from build123d import *

# Parameters (mm, degrees)
F0_W            = 17.96984524
F0_H            = 38.1
F3_DEPTH        = 25.4
F3_COPIES_COUNT = 10


# Not quite as in the source:
# - a pattern or mirror of a feature is missing from the dataset's text; its kind, count and spacing are read off the source's solid


with BuildPart() as f1:
    # F0 (on Front) → F1 (revolve)
    with BuildSketch(Plane.XZ):
        with Locations((-8.98492262, 22.0940720202)):
            Rectangle(F0_W, F0_H)
    revolve(axis=Axis((-8.98492262, 0, 3.0440720202), (1, 0, 0)))

    # F2 (on face) → F3 (cut)
    with BuildSketch(Plane.YZ):
        with BuildLine():
            Line((-6.214665944, 40.6338036926), (-4.1235210374, 31.6734537482))
            Line((-4.1235210374, 31.6734537482), (0, 31.6734537482))
            Line((0, 31.6734537482), (0, 41.1440720202))
            ThreePointArc((0, 41.1440720202), (-3.117789544, 41.0162906591), (-6.214665944, 40.6338036926))
        make_face()
        with BuildLine():
            Line((0, 41.1440720202), (0, 31.6734537482))
            Line((0, 31.6734537482), (4.2036371306, 31.6734537482))
            Line((4.2036371306, 31.6734537482), (6.1898369976, 40.6379002098))
            ThreePointArc((6.1898369976, 40.6379002098), (3.1052492637, 41.0173182208), (0, 41.1440720202))
        make_face()
    f3 = extrude(amount=-F3_DEPTH, mode=Mode.SUBTRACT)

    # F3_copies: F3 ×10 about axis
    f3_copies_axis = Axis((0, 0, 3.044072), (1, 0, 0))
    for i in range(1, F3_COPIES_COUNT):
        add(f3.rotate(f3_copies_axis, i * 360 / F3_COPIES_COUNT), mode=Mode.SUBTRACT)


solid = f1.part
Input: part model. Units: mm. Frame: model coordinates. A direction names the side the tool comes from. Give positions to 0.01 mm unless a question says otherwise; leave off trailing zeros. Order: outer loops, then holes, each group sorted by start corner. A loop starts at its lowest first (then second) coordinate and runs counter-clockwise, first axis right, second up.
Q1. Section D-D on y = -1. Output: boundary loops of the cut face in (x, z), and give its area (3 significant figures).
Checked values:
outline: (-17.97, -25.59) - (0, -25.59) - (0, 31.67) - (-17.97, 31.67) - close
area: 1,030 mm2
Q2. Set-up query: faces 1 (the flat face through (-8.86, -29.95, -12.14)), 2 (the flat face through (-8.859, 33.033, 8.328)), 3 (the flat face through (-8.859, -5.184, 36.216)), 4 (the flat face through (-8.859, 29.947, 18.225)), 5 (the flat face through (-8.86, -23.62, -20.65)). Return all of +Z, -Z, +X, -X, +Y, -Y with unobstructed straight access to the full face (end or side cutting, diameter ignored); none if empty.
Checked values:
face 1: +X, -X, -Y
face 2: +X, -X
face 3: +Z, +X, -X
face 4: +X, -X, +Y
face 5: -Z, +X, -X
Q3. Ray query, probe 1 along Z at (x, y) = (-6.5, -31); probe 2 along Y at (x, z) = (-5.5, 25); probe 3 along Y at (x, z) = (-9.5, -22). Return the intervals inside material, ascending.
Checked values:
probe 1: z = -19.11 to -12.77, -2.04 to 8.18, 18.88 to 25.19
probe 2: y = -31.14 to -21.57, -18.49 to 18.49, 21.66 to 31.14
probe 3: y = -28.71 to -25.15, -14.24 to 14.24, 25.14 to 28.71
Q4. Contact query for flat-ended pins moving along their axis: pin 1 Ø3 at (x, z) = (-4, 29) entering from +Y (3 decimals); pin 2 Ø2.5 at (x, y) = (-7.5, 0.5) entering from +Z; pin 3 Ø5 at (x, z) = (-16, -25) entering from -Y. Output: stop coordinate, or through.
Checked values:
pin 1: stops at y = 29.215
pin 2: stops at z = 31.67
pin 3: stops at y = -28.27
Q5. Section A-A on z = 26. Output: boundary loops of the cut face in (x, y).
Checked values:
outline: (-17.97, -30.41) - (0, -30.41) - (0, -22.73) - (-17.97, -22.73) - close; (-17.97, -17.11) - (0, -17.11) - (0, 17.11) - (-17.97, 17.11) - close; (-17.97, 22.79) - (0, 22.79) - (0, 30.41) - (-17.97, 30.41) - close
Q6. Section C-C on z = -29. Output: boundary loops of the cut face in (x, y), and give its area (3 significant figures).
Checked values:
outline: (-17.97, -16.22) - (0, -16.22) - (0, -4.96) - (-17.97, -4.96) - close; (-17.97, 4.92) - (0, 4.92) - (0, 16.22) - (-17.97, 16.22) - close
area: 405 mm2
Q7. Draft query along Y for faces 6 (the flat face through (-8.86, -5.18, -30)), 7 (the cylindrical face through (-8.86, -11.71, 39.3)), 8 (the cylindrical face through (-8.86, 30.78, -19.41)). Return one class per face: +Y half, -Y half, draft (parallel to the pull), parting line (faces both ways), or undercut.
Checked values:
face 6: undercut
face 7: -Y half
face 8: +Y half
Q8. Section B-B on y = -30.5. Output: boundary loops of the cut face in (x, z).
Checked values:
outline: (-17.97, -19.79) - (0, -19.79) - (0, -12.47) - (-17.97, -12.47) - close; (-17.97, -2) - (0, -2) - (0, 8.14) - (-17.97, 8.14) - close; (-17.97, 18.58) - (0, 18.58) - (0, 25.88) - (-17.97, 25.88) - close
